The model under review builds one solid part; all positions refer to its coordinate system, in mm. Give positions to 0.01 mm unless a question says otherwise; leave off trailing zeros. Write each loop counter-clockwise with the first axis right and the second up, starting at its lowest first coordinate (ties: lowest second). Pieces come first, ordered by that corner, then holes. Notation, with made-up numbers: (76.5, -39) - (90.5, -39) arc R18 ccw to (90.5, -25) - close; hole circle Ø1 at (81.25, 40). An arc over 180 degrees is marked (long way). One line per question, with ' | ' between items. Start each with the question number.
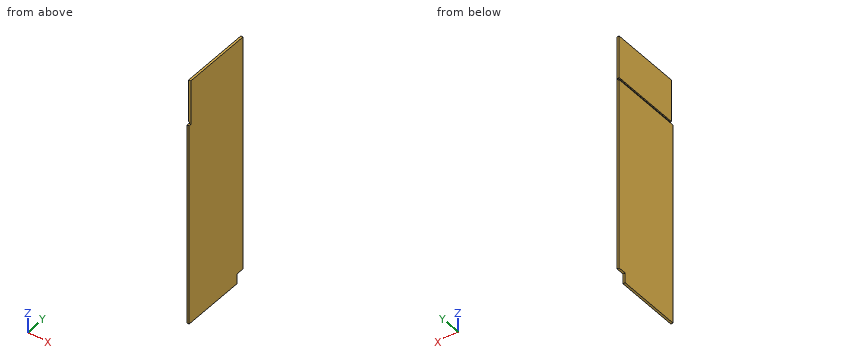
```python
from build123d import *

# Parameters (mm, degrees)
F0_W     = 635
F0_H     = 2231
F1_DEPTH = 19
F2_W     = 9
F2_H     = 19
F3_DEPTH = 635.001
F4_W     = 70
F4_H     = 90
F5_DEPTH = 19.001
F6_W     = 19
F6_H     = 403
F7_DEPTH = 19.001


with BuildPart() as f1:
    # F0 (on Right) → F1 (new body)
    with BuildSketch(Plane.YZ):
        with Locations((317.5, 1115.5)):
            Rectangle(F0_W, F0_H)
    extrude(amount=F1_DEPTH)

    # F2 (on Front) → F3 (cut, through all)
    with BuildSketch(Plane.XZ):
        with Locations((4.5, 1837.5)):
            Rectangle(F2_W, F2_H)
    extrude(amount=-F3_DEPTH, mode=Mode.SUBTRACT)

    # F4 (on Right) → F5 (cut, through all)
    with BuildSketch(Plane.YZ):
        with Locations((600, 45)):
            Rectangle(F4_W, F4_H)
    extrude(amount=F5_DEPTH, mode=Mode.SUBTRACT)

    # F6 (on Right) → F7 (cut, through all)
    with BuildSketch(Plane.YZ):
        with Locations((9.5, 2029.5)):
            Rectangle(F6_W, F6_H)
    extrude(amount=F7_DEPTH, mode=Mode.SUBTRACT)


solid = f1.part
```
Item 1: Take a section at A-A (x = 3.25). Give the boundary of the cut face in (y, z), plus the area to 3 significant figures.
Item 2: For probe 1 along Z at (x, y) = (7, 346.5); probe 2 along Z at (x, y) = (1.25, 589); probe 3 along Y at (x, z) = (10.5, 1889.5), list the stretches that pass through material, from the lowest coordinate up.
Item 3: Clearance check with flat-ended pins moving along their axes: P1, Ø2, axis at x = 11, z = 1901.5, coming from the -Y side; P2, Ø9.5, axis at y = 408.5, z = 1839.5, coming from the -X side. State where each tip first meets the part, or that it passes through.
Item 4: Take a section at B-B (z = 1906). Give the boundary of the cut face in (x, y), plus the area to 3 significant figures.
Check sheet entries:
1) outline: (0, 0) - (565, 0) - (565, 90) - (635, 90) - (635, 1828) - (0, 1828) - close; (19, 1847) - (635, 1847) - (635, 2231) - (19, 2231) - close | area: 1,390,000 mm^2
2) probe 1: z = 0 to 1828, 1847 to 2231 | probe 2: z = 90 to 1828, 1847 to 2231 | probe 3: y = 19 to 635
3) P1: stops at y = 19 | P2: stops at x = 9
4) outline: (0, 19) - (19, 19) - (19, 635) - (0, 635) - close | area: 11,700 mm^2
